Geometry check sheet. Reference: the model listing, model coordinates, mm. Coordinates: 2 decimals unless noted, no trailing zeros. Write each loop counter-clockwise with the first axis right and the second up, starting at its lowest first coordinate (ties: lowest second). Pieces come first, ordered by that corner, then holes. Notation, with made-up numbers: (44, 18.25) - (77, 18.25) arc R8 ccw to (77, 28.25) - close; hole circle Ø3 at (69.25, 38.25). An arc over 180 degrees is marked (long way). Answer as a JSON object with one key per item and string values. Group by question number.
from build123d import *

# Parameters (mm, degrees)
SKETCH1_W           = 25.4
SKETCH1_H           = 190.5
SKETCH1_R           = 3.175
BOSS_EXTRUDE1_DEPTH = 6.35
FILLET2_R           = 12.7
FILLET3_R           = 2.116666667


with BuildPart() as part:
    # Sketch1 → Boss-Extrude1 (new body)
    with BuildSketch(Plane(origin=(0, 0, 0), x_dir=(1, 0, 0), z_dir=(0, 1, 0))):
        Rectangle(SKETCH1_W, SKETCH1_H)
        with Locations(Location((0, -82.55, 0), (0, 0, 270))):
            Circle(SKETCH1_R, mode=Mode.SUBTRACT)
        with Locations(Location((0, 63.5, 0), (0, 0, 270))):
            Circle(SKETCH1_R, mode=Mode.SUBTRACT)
        with Locations(Location((0, 82.55, 0), (0, 0, 270))):
            Circle(SKETCH1_R, mode=Mode.SUBTRACT)
        with Locations(Location((0, -63.5, 0), (0, 0, 270))):
            Circle(SKETCH1_R, mode=Mode.SUBTRACT)
    extrude(amount=BOSS_EXTRUDE1_DEPTH)

    # Fillet2
    fillet2_edges = [part.edges().sort_by_distance(p)[0] for p in [
        (-12.7, 3.175, -95.25),
        (12.7, 3.175, -95.25),
        (-12.7, 3.175, 95.25),
        (12.7, 3.175, 95.25),
    ]]
    fillet(fillet2_edges, radius=FILLET2_R - 0.0001)  # a hair under: the kernel refuses the full size

    # Fillet3
    fillet3_edges = [part.edges().sort_by_distance(p)[0] for p in [
        (-12.7, 0, 0),
        (-12.7, 6.35, 0),
        (12.7, 0, 0),
        (8.98028541, 0, 91.53028541),
        (-8.98028541, 0, 91.53028541),
        (8.98028541, 0, -91.53028541),
        (-8.98028541, 0, -91.53028541),
        (12.7, 6.35, 0),
        (8.98028541, 6.35, 91.53028541),
        (-8.98028541, 6.35, 91.53028541),
        (8.98028541, 6.35, -91.53028541),
        (-8.98028541, 6.35, -91.53028541),
    ]]
    fillet(fillet3_edges, radius=FILLET3_R)


solid = part.part
(1) Section check C-C (z = -23). Record the cut outline in (x, y).
(2) Draft check along X on faces 1 (the face through (0.95, 3.13, 85.58)), 2 (the face through (-9.08, 3.19, -91.43)), 3 (the face through (0, 0, -1)). Enter one of: +X half, -X half, draft (parallel to the pull), parting line (faces both ways), or undercut.
(3) Section check A-A (z = -63.5). Record the cut outline in (x, y) (3 decimals).
(4) Material ranges on L1, parallel to Z at x = 1.5, y = 2; L2, parallel to X at y = 3.25, z = -82.55 (3 decimals); L3, parallel to Z at x = 1.75, y = 4.5, recorded low to high. Write a range as [from, to].
(5) Gauge pin test, flat ends, axial feed: pin 1 (2 mm diameter, centred on y = 1, z = -39, fed in from -X); pin 2 (5 mm diameter, centred on x = 0, z = -63.5, fed in from +Y); pin 3 (1.5 mm diameter, centred on y = 5.5, z = 43.5, fed in from +X). Record the tip position at first contact, or that the pin passes through.
(6) Section check B-B (y = 3.25). Count the separate pieces of the cut face and the enclosed holes in it, and give its area (3 significant figures).
Conclusion:
{
 "1": {"outline": "(-12.7, 2.12) arc R2.12 ccw to (-10.58, 0) - (10.58, 0) arc R2.12 ccw to (12.7, 2.12) - (12.7, 4.23) arc R2.12 ccw to (10.58, 6.35) - (-10.58, 6.35) arc R2.12 ccw to (-12.7, 4.23) - close"},
 "2": {"face 1": "undercut", "face 2": "-X half", "face 3": "draft"},
 "3": {"outline": "(-12.7, 2.117) arc R2.117 ccw to (-10.583, 0) - (-3.175, 0) - (-3.175, 6.35) - (-10.583, 6.35) arc R2.117 ccw to (-12.7, 4.233) - close; (3.175, 0) - (10.583, 0) arc R2.117 ccw to (12.7, 2.117) - (12.7, 4.233) arc R2.117 ccw to (10.583, 6.35) - (3.175, 6.35) - close"},
 "4": {"L1": "z = [-95.16, -85.35], [-79.75, -66.3], [-60.7, 60.7], [66.3, 79.75], [85.35, 95.16]", "L2": "x = [-12.7, -3.175], [3.175, 12.7]", "L3": "z = [-95.11, -85.2], [-79.9, -66.15], [-60.85, 60.85], [66.15, 79.9], [85.2, 95.11]"},
 "5": {"pin 1": "stops at x = -12.7", "pin 2": "passes through", "pin 3": "stops at x = 12.64"},
 "6": {"separate pieces": "1", "enclosed holes": "4", "area": "4,570 mm^2"}
}
